Verification items for the finished model (mm, model axes). A direction names the side the tool comes from. Give positions to 0.01 mm unless a question says otherwise; leave off trailing zeros. Order: outer loops, then holes, each group sorted by start corner. A loop starts at its lowest first (then second) coordinate and runs counter-clockwise, first axis right, second up.
(1) Sectioned sample at B-B on x = 0. Record the cut outline in (y, z), plus the area to 3 significant figures.
(2) Sectioned sample at D-D on z = 89.5. Record the cut outline in (x, y), plus the area to 3 significant figures.
(3) Sectioned sample at A-A on y = -4.5. Record the cut outline in (x, z), plus the area to 3 significant figures.
(4) Sectioned sample at C-C on z = 35. Record the cut outline in (x, y), plus the area to 3 significant figures.
(5) Scan lines: L1, parallel to X at y = -13.5, z = 62; L2, parallel to X at y = 0.5, z = 19.5; L3, parallel to Y at x = 0, z = 11. Record each from-to range of solid material in increasing order.
(6) Access from +Z, -Z, +X, -X, +Y, -Y to the whole of each face (thin tool, end or side, straight path). Record for faces 1 (the face through (-55, 0, 71)), 2 (the face through (-60.07, 0.33, 72.507)).
(7) Mould release check, pull along Y, two halves, no side actions. Record for faces 3 (the face through (-60.07, -0.55, 104.994)), 4 (the face through (14.985, 0.66, 24.65)), 5 (the face through (55, 0, 72)): pulls with the +Y half, pulls with the -Y half, needs draft (parallel to the pull), parting line crosses it, or undercut.
(8) Gauge pin test, flat ends, axial feed: pin 1 (10 mm diameter, centred on x = -2.5, y = 6.5, fed in from +Z); pin 2 (1 mm diameter, centred on x = 42, y = 15.5, fed in from +Z). Record the tip position at first contact, or that the pin passes through.
Autodesk Inventor part; units mm, degrees
ref_plane "YZ Plane" through (0, 0, 0) normal (1, 0, 0) x (0, 1, 0)
ref_plane "XZ Plane" through (0, 0, 0) normal (0, 1, 0) x (-1, 0, 0)
ref_plane "XY Plane" through (0, 0, 0) normal (0, 0, 1) x (1, 0, 0)
sketch "Boceto1" plane through (0, 0, 0) normal (0, 0, 1) x (1, 0, 0)
  line L0 (65, -25) -> (-65, -25)
  line L1 (-65, -25) -> (-65, 25)
  line L2 (-65, 25) -> (65, 25)
  line L3 (65, 25) -> (65, -25)
  line L4 (65, -25) -> (-65, 25) construction
  line L5 (-65, -25) -> (65, 25) construction
  point P0 (0, 0)
  dimension "d0" = 130
  dimension "d1" = 50
extrude "Extrusión1" add sketch "Boceto1" along normal blind 50
sketch "Boceto2" plane through (65, -25, 0) normal (1, 0, 0) x (0, 0, -1)
  line L0 (-50, 0) -> (-80, 0)
  line L1 (-50, 0) -> (-50, 50)
  line L2 (-50, 50) -> (-80, 50)
  arc A0 (-80, 50) -> (-80, 0) centre (-80, 25) ccw
  circle A1 centre (-80, 25) radius 7.5
  point P0 (0, 25)
  dimension "d4" = 30
  dimension "d5" = 30
  dimension "d6" = 15
extrude "Extrusión2" add sketch "Boceto2" against normal blind 10
sketch "Boceto3" plane through (-65, -25, 0) normal (-1, 0, 0) x (0, 0, 1)
  circle A0 centre (80, 25) radius 7.5
  arc A1 (80, 0) -> (80, 50) centre (80, 25) ccw
  line L0 (80, 50) -> (50, 50)
  line L1 (50, 50) -> (50, 0)
  line L2 (50, 0) -> (80, 0)
  point P0 (0, 25)
extrude "Extrusión3" add sketch "Boceto3" against normal blind 10
sketch "Boceto4" plane through (0, 0, 0) normal (0, 0, -1) x (-1, 0, 0)
  circle A0 centre (0, 0) radius 15
  dimension "d11" = 30
extrude "Extrusión4" cut sketch "Boceto4" against normal up to next
properties part number "Muñeca"
Ans:
1. outline: (-25, 0) - (-15, 0) - (-15, 50) - (-25, 50) - close; (15, 0) - (25, 0) - (25, 50) - (15, 50) - close
1. area: 1,000 mm2
2. outline: (-65, -23.12) - (-55, -23.12) - (-55, 23.12) - (-65, 23.12) - close; (55, -23.12) - (65, -23.12) - (65, 23.12) - (55, 23.12) - close
2. area: 925 mm2
3. outline: (-65, 0) - (-14.31, 0) - (-14.31, 50) - (-55, 50) - (-55, 74) - (-65, 74) - close; (-65, 86) - (-55, 86) - (-55, 104.59) - (-65, 104.59) - close; (14.31, 0) - (65, 0) - (65, 74) - (55, 74) - (55, 50) - (14.31, 50) - close; (55, 86) - (65, 86) - (65, 104.59) - (55, 104.59) - close
3. area: 5,920 mm2
4. outline: (-65, -25) - (65, -25) - (65, 25) - (-65, 25) - close; hole circle Ø30 at (0, 0)
4. area: 5,790 mm2
5. L1: x = -65 to -55, 55 to 65
5. L2: x = -65 to -14.99, 14.99 to 65
5. L3: y = -25 to -15, 15 to 25
6. face 1: +Z, +Y, -Y
6. face 2: +X, -X
7. face 3: parting line crosses it
7. face 4: undercut
7. face 5: needs draft
8. pin 1: passes through
8. pin 2: stops at z = 50
